```python
from build123d import *

# Parameters (mm, degrees)
F0_W      = 101.6
F0_H      = 60.33
F1_DEPTH  = 12.7
F3_DEPTH  = 101.6
F4_W      = 13.7607939541
F4_H      = 10.2049419656
F5_DEPTH  = 3.175
F6_DEPTH  = 3.175
F7_W      = 0.254
F7_H      = 12.7
F8_DEPTH  = 101.6
F10_DEPTH = 25.4
F11_W     = 0.7027839153
F11_H     = 7.62
F14_W     = 24.6972160847
F14_H     = 5.7475257993
F15_DEPTH = 7.62
F17_DEPTH = 6.35


with BuildPart() as f1:
    # F0 (on Front) → F1 (new body)
    with BuildSketch(Plane.XZ):
        with Locations((50.8, 30.165)):
            Rectangle(F0_W, F0_H)
    extrude(amount=F1_DEPTH)

    # F2 (on face) → F3 (join)
    with BuildSketch(Plane.YZ.offset(101.6)):
        Polygon((0, -7.62), (-2.7734531851, 0), (-9.9265468149, 0), (-12.7, -7.62), align=None)
    extrude(amount=-F3_DEPTH)

    # F4 (on face) → F5 (cut)
    with BuildSketch(Plane(origin=(0, 0, 0), x_dir=(0, -1, 0), z_dir=(-1, 0, 0))):
        with Locations((6.8803969771, -5.1024709828)):
            Rectangle(F4_W, F4_H)
    extrude(amount=-F5_DEPTH, mode=Mode.SUBTRACT)

    # F6 (add): a face of the model
    f6_faces = [f1.faces().sort_by_distance(p)[0] for p in [
        (3.175, -6.35, -4.1648349301),
    ]]
    extrude(f6_faces, amount=F6_DEPTH)

    # F7 (on face) → F8 (cut)
    with BuildSketch(Plane.XY.offset(60.33)):
        with Locations((101.473, -6.35)):
            Rectangle(F7_W, F7_H)
    extrude(amount=-F8_DEPTH, mode=Mode.SUBTRACT)

    # F9 (on face) → F10 (cut)
    with BuildSketch(Plane.YZ.offset(101.346)):
        Polygon((-9.9265468149, 0), (-12.7, -7.62), (0, -7.62), (-2.7734531851, 0), align=None)
    extrude(amount=-F10_DEPTH, mode=Mode.SUBTRACT)

    # F13: sweep along a path in F12
    with BuildLine(Plane(origin=(0, 0, 0), x_dir=(1, 0, 0), z_dir=(0, 0, -1))) as f13_path:
        Line((75.946, 9.9265468149), (101.346, 9.9265468149))
        Line((101.346, 9.9265468149), (101.346, 2.7734531851))
        Line((101.346, 2.7734531851), (75.946, 2.7734531851))
    # F11 (on face) → F13 (sweep)
    with BuildSketch(Plane.YZ.offset(75.946)):
        Polygon((-9.9265468149, 0), (-12.7, -7.62), (-9.9265468149, -7.62), align=None)
        with Locations((-9.5751548573, -3.81)):
            Rectangle(F11_W, F11_H)
    sweep(path=f13_path.line, transition=Transition.RIGHT)

    # F14 (on face) → F15 (join)
    with BuildSketch(Plane(origin=(0, 0, -7.62), x_dir=(1, 0, 0), z_dir=(0, 0, -1))):
        with Locations((88.2946080424, 6.35)):
            Rectangle(F14_W, F14_H)
    extrude(amount=-F15_DEPTH)

    # F16 (on face) → F17 (join)
    with BuildSketch(Plane(origin=(0, 0, 0), x_dir=(0, -1, 0), z_dir=(-1, 0, 0))):
        with BuildLine():
            ThreePointArc((8.89, 43.18), (6.35, 45.72), (3.81, 43.18))
            Line((3.81, 43.18), (8.89, 43.18))
        make_face()
        with BuildLine():
            Line((8.89, 43.18), (3.81, 43.18))
            ThreePointArc((3.81, 43.18), (6.35, 40.64), (8.89, 43.18))
        make_face()
        with BuildLine():
            Line((8.89, 17.145), (3.81, 17.145))
            ThreePointArc((3.81, 17.145), (6.35, 14.605), (8.89, 17.145))
        make_face()
        with BuildLine():
            ThreePointArc((8.89, 17.145), (6.35, 19.685), (3.81, 17.145))
            Line((3.81, 17.145), (8.89, 17.145))
        make_face()
    extrude(amount=F17_DEPTH)


solid = f1.part
```
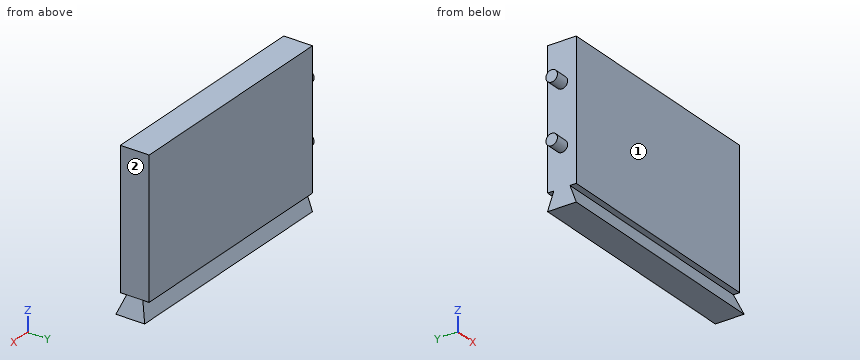
The model under review builds one solid part; all positions refer to its coordinate system, in mm. Face numbers are marked on the shaded views. A direction names the side the tool comes from. Round coordinates to 2 decimals unless told otherwise and drop trailing zeros. Order: outer loops, then holes, each group sorted by start corner. A loop starts at its lowest first (then second) coordinate and runs counter-clockwise, first axis right, second up. Notation, with made-up numbers: (7, 14.25) - (16, 14.25) arc R24 ccw to (16, 24.25) - close; hole circle Ø3 at (-15, 2). An arc over 180 degrees is marked (long way). Answer in a Markdown table with one row per item.
(1) Take a section at A-A on x = 52. Write out the cut boundary in (y, z), plus the area to 3 significant figures.
Result set:
| item | result |
|---|---|
| outline | (-12.7, -7.62) - (0, -7.62) - (-2.77, 0) - (0, 0) - (0, 60.33) - (-12.7, 60.33) - (-12.7, 0) - (-9.93, 0) - close |
| area | 842 mm2 |
(2) For line 1 (X direction, y = -6.75, z = 17.5); line 2 (X direction, y = -6.25, z = 22); line 3 (Y direction, x = 15.5, z = -1), list the stretches that pass through material, from the lowest coordinate up. Write a range as from..to.
Result set:
| item | result |
|---|---|
| line 1 | x = -6.35..101.35 |
| line 2 | x = 0..101.35 |
| line 3 | y = -10.29..-2.41 |
(3) Take a section at C-C on z = 43.18. Write out the cut boundary in (x, y), plus the area to 3 significant figures.
Result set:
| item | result |
|---|---|
| outline | (-6.35, -8.89) - (0, -8.89) - (0, -12.7) - (101.35, -12.7) - (101.35, 0) - (0, 0) - (0, -3.81) - (-6.35, -3.81) - close |
| area | 1,320 mm2 |
(4) Machinability: for the marked faces 1 and 2, which of the approach directions +Z, -Z, +X, -X, +Y, -Y give a long, thin tool a straight path to every point of the face, cutting with its end or side? Answer none if there is none.
Result set:
| item | result |
|---|---|
| face 1 | +Z, -Z, +X, -X, -Y |
| face 2 | +Z, +X, +Y, -Y |
(5) Clearance check with flat-ended pins moving along their axes: P1, Ø1, axis at y = -5, z = 15.5, coming from the +X side; P2, Ø2, axis at y = -2.5, z = 14, coming from the -X side. State where each tip first meets the part, or that it passes through.
Result set:
| item | result |
|---|---|
| P1 | stops at x = 101.35 |
| P2 | stops at x = 0 |
(6) Take a section at B-B on y = -6.35. Write out the cut boundary in (x, z) (3 decimals), plus the area to 3 significant figures.
Result set:
| item | result |
|---|---|
| outline | (-6.35, 14.605) - (0, 14.605) - (0, -7.62) - (104.119, -7.62) - (101.346, 0) - (101.346, 60.33) - (0, 60.33) - (0, 45.72) - (-6.35, 45.72) - (-6.35, 40.64) - (0, 40.64) - (0, 19.685) - (-6.35, 19.685) - close |
| area | 6,960 mm2 |
(7) Take a section at D-D on z = 4.5. Write out the cut boundary in (x, y), plus the area to 3 significant figures.
Result set:
| item | result |
|---|---|
| outline | (0, -12.7) - (101.35, -12.7) - (101.35, 0) - (0, 0) - close |
| area | 1,290 mm2 |
